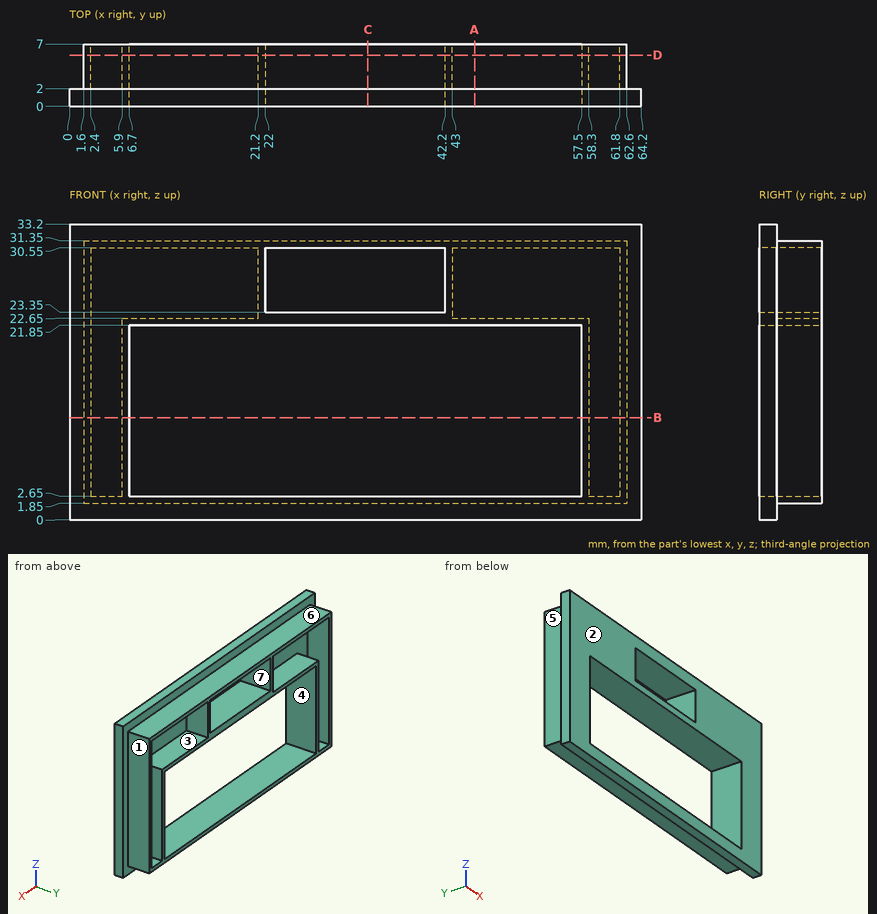
Verification items for this drawing (mm, ordinates from the low corner). A direction names the side the tool comes from. Coordinates: 2 decimals unless noted, no trailing zeros. Order: outer loops, then holes, each group sorted by start corner. A loop starts at its lowest first (then second) coordinate and runs counter-clockwise, first axis right, second up. Notation, with made-up numbers: (-19.75, 37) -> (-0.75, 37) arc R32 ccw to (-0.75, 65) -> close; hole circle Ø1 at (-35, -8.75). An arc over 180 degrees is marked (long way). Answer as CSV lines item,"result". Start each with the question number.
1) Cross-section at D-D, the plane y = 5.75. Record the boundary of the cut face in (x, z).
2) Set-up check for the marked faces 1, 2, 3 and 4: record each of +Z, -Z, +X, -X, +Y, -Y from which the full face is reachable in a straight line by a thin tool's end or side.
3) Cross-section at B-B, the plane z = 11.5. Record the boundary of the cut face in (x, y), then the cut area to 3 significant figures.
4) Release check for a two-part mould opening along Z. For the marked faces 5, 6 and 7 record: released by +Z, released by -Z, zero draft, split by the parting line, or undercut.
5) Gauge pin test, flat ends, axial feed: pin 1 Ø2.5 at (y, z) = (3.5, 27.5) entering from +X; pin 2 Ø2 at (y, z) = (4, 26.5) entering from -X; pin 3 Ø5 at (x, z) = (46, 7.5) entering from -Y; pin 4 Ø16.5 at (x, z) = (40.5, 18) entering from +Y. Record the tip position at first contact, or that the pin passes through.
6) Material ranges on L1, parallel to X at y = 4, z = 12; L2, parallel to Z at x = 44, y = 5.5; L3, parallel to Z at x = 32, y = 6.75, recorded low to high. Write a range as [from, to].
7) Cross-section at A-A, the plane x = 45.5. Record the boundary of the cut face in (y, z).
8) Cross-section at C-C, the plane x = 33.5. Record the boundary of the cut face in (y, z), then the cut area to 3 significant figures.
Conclusion:
1,outline,"(1.6, 1.85) -> (62.6, 1.85) -> (62.6, 31.35) -> (1.6, 31.35) -> close; hole (2.4, 2.65) -> (5.9, 2.65) -> (5.9, 22.65) -> (21.2, 22.65) -> (21.2, 30.55) -> (2.4, 30.55) -> close; hole (6.7, 2.65) -> (57.5, 2.65) -> (57.5, 21.85) -> (6.7, 21.85) -> close; hole (22, 23.35) -> (42.2, 23.35) -> (42.2, 30.55) -> (22, 30.55) -> close; hole (43, 22.65) -> (58.3, 22.65) -> (58.3, 2.65) -> (61.8, 2.65) -> (61.8, 30.55) -> (43, 30.55) -> close"
2,face 1,"+Z, -Z, +X, +Y"
2,face 2,"+Z, -Z, +X, -X, -Y"
2,face 3,"+Y"
2,face 4,"+Y, -Y"
3,outline,"(0, 0) -> (6.7, 0) -> (6.7, 7) -> (5.9, 7) -> (5.9, 2) -> (2.4, 2) -> (2.4, 7) -> (1.6, 7) -> (1.6, 2) -> (0, 2) -> close; (57.5, 0) -> (64.2, 0) -> (64.2, 2) -> (62.6, 2) -> (62.6, 7) -> (61.8, 7) -> (61.8, 2) -> (58.3, 2) -> (58.3, 7) -> (57.5, 7) -> close"
3,area,"42.8 mm²"
4,face 5,"zero draft"
4,face 6,"released by +Z"
4,face 7,"undercut"
5,pin 1,"stops at x = 62.6"
5,pin 2,"stops at x = 1.6"
5,pin 3,"passes through"
5,pin 4,"stops at y = 7"
6,L1,"x = [1.6, 2.4], [5.9, 6.7], [57.5, 58.3], [61.8, 62.6]"
6,L2,"z = [1.85, 2.65], [21.85, 22.65], [30.55, 31.35]"
6,L3,"z = [1.85, 2.65], [21.85, 23.35], [30.55, 31.35]"
7,outline,"(0, 0) -> (2, 0) -> (2, 1.85) -> (7, 1.85) -> (7, 2.65) -> (0, 2.65) -> close; (0, 21.85) -> (7, 21.85) -> (7, 22.65) -> (2, 22.65) -> (2, 30.55) -> (7, 30.55) -> (7, 31.35) -> (2, 31.35) -> (2, 33.2) -> (0, 33.2) -> close"
8,outline,"(0, 0) -> (2, 0) -> (2, 1.85) -> (7, 1.85) -> (7, 2.65) -> (0, 2.65) -> close; (0, 21.85) -> (7, 21.85) -> (7, 23.35) -> (0, 23.35) -> close; (0, 30.55) -> (7, 30.55) -> (7, 31.35) -> (2, 31.35) -> (2, 33.2) -> (0, 33.2) -> close"
8,area,"29.1 mm²"
